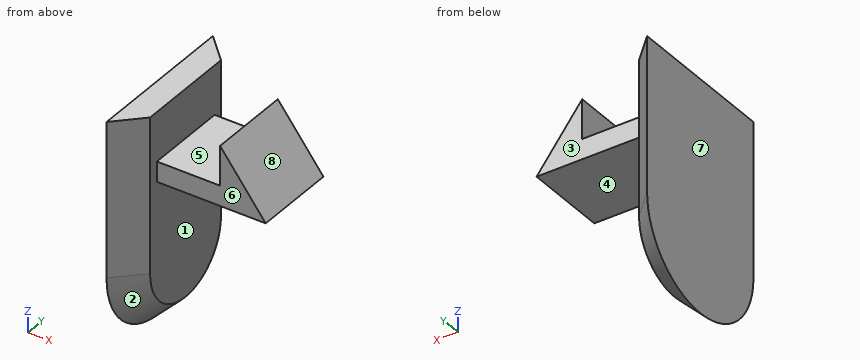
from build123d import *

# Parameters (mm, degrees)
F0_W     = 12
F0_H     = 18
F1_DEPTH = 2
F3_R     = 5.99999
F4_SIZE  = 1.99999
F5_W     = 6.5143028369
F5_H     = 4.6212589368
F6_DEPTH = 10
F7_W     = 4.9025638513
F7_H     = 3.0622794293
F8_DEPTH = 25


# Not quite as in the source:
# - a fillet or chamfer is up to 0.001 mm smaller than in the source, because OpenCascade refuses the exact size


with BuildPart() as f1:
    # F0 (on Right) → F1 (new body)
    with BuildSketch(Plane.YZ):
        Rectangle(F0_W, F0_H)
    extrude(amount=F1_DEPTH)

    # F3 (radius 6 in the source; OpenCascade refuses exactly that, so slightly less here)
    f3_edges = [f1.edges().sort_by_distance(p)[0] for p in [
        (1, 6, -9),
        (1, -6, -9),
    ]]
    fillet(f3_edges, radius=F3_R)

    # F4 (size 2 in the source; OpenCascade refuses exactly that, so slightly less here)
    f4_edges = [f1.edges().sort_by_distance(p)[0] for p in [
        (2, 4.242644, -7.242644),
        (2, -6, 2.999995),
    ]]
    chamfer(f4_edges, length=F4_SIZE)

    # F5 (on face) → F6 (join)
    with BuildSketch(Plane.YZ.offset(2)):
        with Locations((0.0278381212, 5.9414044954)):
            Rectangle(F5_W, F5_H)
    extrude(amount=F6_DEPTH)

    # F7 (on face) → F8 (cut)
    with BuildSketch(Plane.XZ.offset(3.2293132972)):
        Polygon((6.9025638513, 9.0315220878), (6.9025638513, 8.2520339638), (10.911365971, 3.0183200724), (13.6395776644, 3.0183200724), (12.8879277036, 9.0315220878), align=None)
        with Locations((4.4512819257, 6.7208942492)):
            Rectangle(F7_W, F7_H)
    extrude(amount=-F8_DEPTH, mode=Mode.SUBTRACT)


solid = f1.part
The model under review builds one solid part; all positions refer to its coordinate system, in mm. Face numbers are marked on the shaded views. A direction names the side the tool comes from. Round coordinates to 2 decimals unless told otherwise and drop trailing zeros. Write each loop counter-clockwise with the first axis right and the second up, starting at its lowest first coordinate (ties: lowest second). Pieces come first, ordered by that corner, then holes. Notation, with made-up numbers: M 21,72 L 41,72 A24 cw 41,94 Z; hole C 31,42.5 d8. An arc over 180 degrees is marked long. Use a Markdown table: item, result. Add a question column.
Q1. Insertion check: pin 1 (2.5 mm diameter, centred on y = 1, z = 4.5, fed in from +X); pin 2 (1.5 mm diameter, centred on x = 3, y = 1.5, fed in from -Z); pin 3 (2.5 mm diameter, centred on x = 4, y = 0, fed in from +Z). Each pin has a flat end and moves straight along its axis. Give the tip position at first contact, or say it passes through.
Q2. To check wall thickness, follow line 1 (Z direction, x = 5.25, y = 0.5); line 2 (X direction, y = -0.75, z = -1.5); line 3 (X direction, y = 2.5, z = 5.5). State the ranges of each line that lie inside material, in increasing order.
Q3. The part is to be moulded in two halves that separate along X. For the marked faces 1, 2 and 3, say which applies: pulls with the +X half, pulls with the -X half, needs draft (parallel to the pull), parting line crosses it, or undercut.
Q4. We need section B-B, the plane x = 3.75. State the section outline as (y, z) points, plus the area to 3 significant figures.
Q5. Machinability: for the marked faces 4, 5, 6, 7 and 8, which of the approach directions +Z, -Z, +X, -X, +Y, -Y give a long, thin tool a straight path to every point of the face, cutting with its end or side? Answer none if there is none.
Findings below:
| question | item | result |
|---|---|---|
| 1 | pin 1 | stops at x = 10.44 |
| 1 | pin 2 | stops at z = 3.63 |
| 1 | pin 3 | stops at z = 5.19 |
| 2 | line 1 | z = 3.63 to 5.19 |
| 2 | line 2 | x = 0 to 2 |
| 2 | line 3 | x = 0 to 2, 6.9 to 9.01 |
| 3 | face 1 | undercut |
| 3 | face 2 | pulls with the +X half |
| 3 | face 3 | needs draft |
| 4 | outline | M -3.23,3.63 L 3.28,3.63 L 3.28,5.19 L -3.23,5.19 Z |
| 4 | area | 10.2 mm² |
| 5 | face 4 | -Z, +X, +Y, -Y |
| 5 | face 5 | +Z, +Y, -Y |
| 5 | face 6 | +Z, -Z, +X, -Y |
| 5 | face 7 | +Z, -Z, -X, +Y, -Y |
| 5 | face 8 | +Z, +X, +Y, -Y |
